Work out the finished part from the listing and answer in its coordinate system (mm). A direction names the side the tool comes from. Round coordinates to 2 decimals unless told otherwise and drop trailing zeros. Order: outer loops, then holes, each group sorted by start corner. A loop starts at its lowest first (then second) coordinate and runs counter-clockwise, first axis right, second up. Notation, with made-up numbers: (88, 25.25) -> (94, 25.25) arc R17 ccw to (94, 49.25) -> close; hole circle Ø6 at (59, 46). An arc over 180 degrees is marked (long way). Use a Markdown table: item, result. Add a question column.
Item 1: A cutting plane is placed at B-B, the plane z = 1.3. Determine the outline of the cut face in (x, y).
Item 2: A cutting plane is placed at C-C, the plane x = 25.5. Determine the outline of the cut face in (y, z), plus the area to 3 significant figures.
Item 3: Find the intervals of material crossed by L1, parallel to X at y = 5, z = 1.55; L2, parallel to Y at x = 24.5, z = 0.25, in increasing order. Write a range as [from, to].
Item 4: A tool of negligible diameter and unlimited length cuts with its end or side. For faces 5 (the flat face through (-35, -23, 1)), 6 (the flat face through (-40, 2, 1)), 7 (the flat face through (13, 29, 1)), 8 (the flat face through (-36, 28, 1)), from which of +Z, -Z, +X, -X, +Y, -Y can it reach the whole face along a straight path? Write none if from no direction.
Item 5: For a pull along X with two mould halves and no side action, classify faces 1 (the flat face through (-44, 3, 1)), 2 (the flat face through (-17, -24, 1)), 3 (the flat face through (40, 2, 1)), 4 (the flat face through (-22, -25, 1)) as +X half, -X half, draft (parallel to the pull), parting line (faces both ways), or undercut.
Item 6: A cutting plane is placed at A-A, the plane y = -1. Determine the outline of the cut face in (x, z), plus the area to 3 significant figures.
Item 7: Flat-ended cylindrical pins translate along their axes: P1, Ø1, axis at x = -41.5, z = 1, coming from the +Y side; P2, Ø0.6, axis at y = -23.5, z = 1, coming from the -X side. Find the tip coordinate at first contact, or state that the pin passes through.
Solid Edge part; units mm, degrees
sketch "Sketch1" plane through (0, 0, 0) normal (0, 0, 1) x (1, 0, 0)
  line L0 (40, -25) -> (40, 30)
  line L1 (40, 30) -> (-44, 30)
  line L2 (-44, 30) -> (-44, -25)
  line L3 (-44, -25) -> (40, -25)
extrude "ExtrudedProtrusion_3" add sketch "Sketch1" along normal blind 2
sketch "Sketch2" plane through (0, 0, 0) normal (0, 0, 1) x (1, 0, 0)
  line L0 (-44, 28) -> (-27, 28)
  line L1 (-27, 28) -> (-27, 30)
  line L2 (-27, 30) -> (-44, 30)
  line L3 (-44, 30) -> (-44, 28)
extrude "ExtrudedCutout_9" cut sketch "Sketch2" along normal blind 2
sketch "Sketch3" plane through (0, 0, 0) normal (0, 0, 1) x (1, 0, 0)
  line L0 (-17, 28) -> (13, 28)
  line L1 (13, 28) -> (13, 30)
  line L2 (13, 30) -> (-17, 30)
  line L3 (-17, 30) -> (-17, 28)
extrude "ExtrudedCutout_10" cut sketch "Sketch3" along normal blind 2
sketch "Sketch4" plane through (0, 0, 0) normal (0, 0, 1) x (1, 0, 0)
  line L0 (23, 28) -> (40, 28)
  line L1 (40, 28) -> (40, 30)
  line L2 (40, 30) -> (23, 30)
  line L3 (23, 30) -> (23, 28)
extrude "ExtrudedCutout_11" cut sketch "Sketch4" along normal blind 2
sketch "Sketch5" plane through (0, 0, 0) normal (0, 0, 1) x (1, 0, 0)
  line L0 (38, -2.5) -> (38, 7.5)
  line L1 (38, 7.5) -> (36, 7.5)
  line L2 (36, 7.5) -> (36, -2.5)
  line L3 (36, -2.5) -> (38, -2.5)
extrude "ExtrudedCutout_12" cut sketch "Sketch5" along normal blind 2
sketch "Sketch6" plane through (0, 0, 0) normal (0, 0, 1) x (1, 0, 0)
  line L0 (40, -23) -> (23, -23)
  line L1 (23, -23) -> (23, -25)
  line L2 (23, -25) -> (40, -25)
  line L3 (40, -25) -> (40, -23)
extrude "ExtrudedCutout_13" cut sketch "Sketch6" along normal blind 2
sketch "Sketch7" plane through (0, 0, 0) normal (0, 0, 1) x (1, 0, 0)
  line L0 (13, -23) -> (-17, -23)
  line L1 (-17, -23) -> (-17, -25)
  line L2 (-17, -25) -> (13, -25)
  line L3 (13, -25) -> (13, -23)
extrude "ExtrudedCutout_14" cut sketch "Sketch7" along normal blind 2
sketch "Sketch8" plane through (0, 0, 0) normal (0, 0, 1) x (1, 0, 0)
  line L0 (-27, -23) -> (-44, -23)
  line L1 (-44, -23) -> (-44, -25)
  line L2 (-44, -25) -> (-27, -25)
  line L3 (-27, -25) -> (-27, -23)
extrude "ExtrudedCutout_15" cut sketch "Sketch8" along normal blind 2
sketch "Sketch9" plane through (0, 0, 0) normal (0, 0, 1) x (1, 0, 0)
  line L0 (-40, -2.5) -> (-40, 7.5)
  line L1 (-40, 7.5) -> (-42, 7.5)
  line L2 (-42, 7.5) -> (-42, -2.5)
  line L3 (-42, -2.5) -> (-40, -2.5)
extrude "ExtrudedCutout_16" cut sketch "Sketch9" along normal blind 2
properties material "Acrylic, high impact grade"
Reported:
| question | item | result |
|---|---|---|
| 1 | outline | (-44, -23) -> (-27, -23) -> (-27, -25) -> (-17, -25) -> (-17, -23) -> (13, -23) -> (13, -25) -> (23, -25) -> (23, -23) -> (40, -23) -> (40, 28) -> (23, 28) -> (23, 30) -> (13, 30) -> (13, 28) -> (-17, 28) -> (-17, 30) -> (-27, 30) -> (-27, 28) -> (-44, 28) -> close; hole (-42, -2.5) -> (-40, -2.5) -> (-40, 7.5) -> (-42, 7.5) -> close; hole (36, -2.5) -> (38, -2.5) -> (38, 7.5) -> (36, 7.5) -> close |
| 2 | outline | (-23, 0) -> (28, 0) -> (28, 2) -> (-23, 2) -> close |
| 2 | area | 102 mm² |
| 3 | L1 | [-44, -42], [-40, 36], [38, 40] |
| 3 | L2 | [-23, 28] |
| 4 | face 5 | +Z, -Z, -X, -Y |
| 4 | face 6 | +Z, -Z |
| 4 | face 7 | +Z, -Z, +Y |
| 4 | face 8 | +Z, -Z, -X, +Y |
| 5 | face 1 | -X half |
| 5 | face 2 | undercut |
| 5 | face 3 | +X half |
| 5 | face 4 | draft |
| 6 | outline | (-44, 0) -> (-42, 0) -> (-42, 2) -> (-44, 2) -> close; (-40, 0) -> (36, 0) -> (36, 2) -> (-40, 2) -> close; (38, 0) -> (40, 0) -> (40, 2) -> (38, 2) -> close |
| 6 | area | 160 mm² |
| 7 | P1 | y = 28 |
| 7 | P2 | x = -27 |
